Design review of the part shown in the three views and the two pictorial views. Dimensions are in mm from the part's minimum x, y and z. A direction names the side the tool comes from. Coordinates: 2 decimals unless noted, no trailing zeros. Loops run counter-clockwise (first coordinate to the right, second up) from the corner with the lowest first, then second, coordinate; pieces in that order, holes last. Notation, with made-up numbers: (20.5, 41.5) -> (73.5, 41.5) arc R17 ccw to (73.5, 53.5) -> close; hole circle Ø11 at (49, 32.5). An arc over 180 degrees is marked (long way). One line per item, written item: value. Start each with the question number.
1. For probe 1 along X at (y, z) = (4, 8); probe 2 along Z at (x, y) = (10, 7.75); probe 3 along Y at (x, z) = (95.5, 14.5), list the stretches that pass through material, from the lowest coordinate up.
2. Machinability: for the marked faces 1, 2 and 3, which of the approach directions +Z, -Z, +X, -X, +Y, -Y give a long, thin tool a straight path to every point of the face, cutting with its end or side? Answer none if there is none.
3. Add section B-B on x = 116.5. Write out the cut boundary in (y, z), plus the area to 3 significant figures.
4. Add section D-D on y = 31. Write out the cut boundary in (x, z), plus the area to 3 significant figures.
5. Insertion check: pin 1 (4 mm diameter, centred on x = 105, z = 6, fed in from +Y); pin 2 (6 mm diameter, centred on x = 118, z = 6.5, fed in from +Y); pin 3 (4 mm diameter, centred on x = 75.5, z = 10, fed in from -Y); pin 4 (2.5 mm diameter, centred on y = 23.5, z = 5.5, fed in from +X). Each pin has a flat end and moves straight along its axis. Give the tip position at first contact, or say it passes through.
6. Add section A-A on z = 8. Give the number of separate pieces and of enclosed holes in the cut face, plus the area to 3 significant figures.
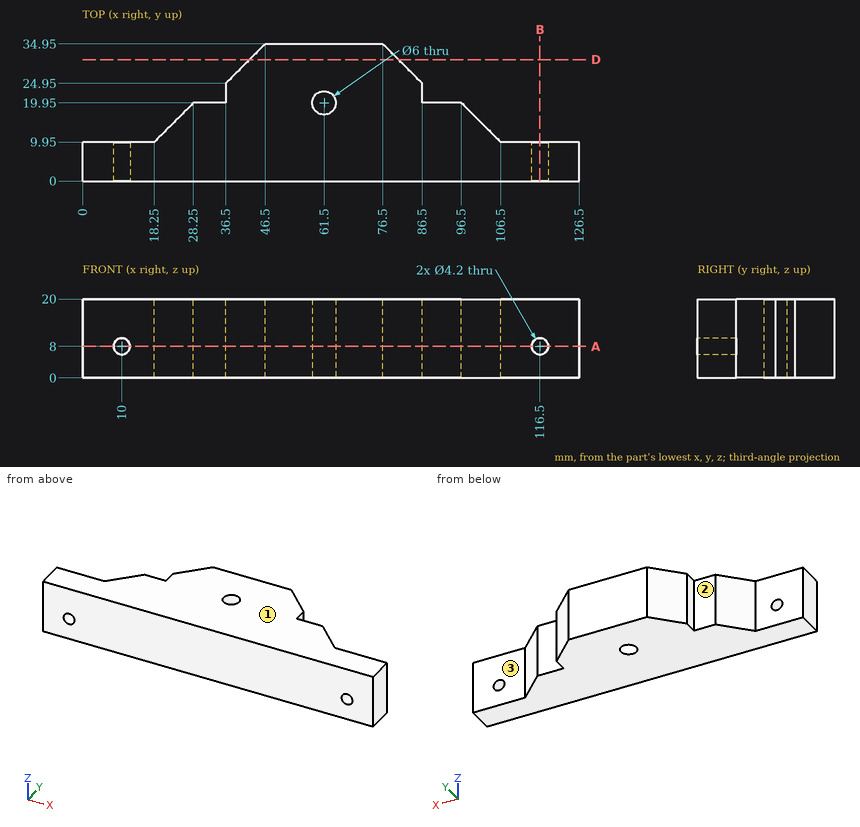
Worked answers:
1. probe 1: x = 0 to 7.9, 12.1 to 114.4, 118.6 to 126.5
1. probe 2: z = 0 to 5.9, 10.1 to 20
1. probe 3: y = 0 to 19.95
2. face 1: +Z, +X, -X, +Y, -Y
2. face 2: +Z, -Z, -X, +Y
2. face 3: +Z, -Z, +X, +Y
3. outline: (0, 0) -> (9.95, 0) -> (9.95, 5.9) -> (0, 5.9) -> close; (0, 10.1) -> (9.95, 10.1) -> (9.95, 20) -> (0, 20) -> close
3. area: 157 mm²
4. outline: (42.55, 0) -> (80.45, 0) -> (80.45, 20) -> (42.55, 20) -> close
4. area: 758 mm²
5. pin 1: stops at y = 13.45
5. pin 2: stops at y = 9.95
5. pin 3: stops at y = 0
5. pin 4: stops at x = 86.5
6. separate pieces: 3
6. enclosed holes: 1
6. area: 2,580 mm²
